Read the model definition and answer for the solid it produces. Units are mm, in the model's axes. Coordinates: 2 decimals unless noted, no trailing zeros. Write each loop counter-clockwise with the first axis right and the second up, starting at its lowest first coordinate (ties: lowest second). Pieces come first, ordered by that corner, then holes. Notation, with made-up numbers: M -38.75,27 L 19.25,27 A21 ccw 19.25,56 Z; hole C 61,25 d5. An arc over 180 degrees is marked long. Use a Markdown table: item, result. Add a question column.
from build123d import *

# Parameters (mm, degrees)
SKETCH1_R                  = 12.5
BOSS_EXTRUDE1_DEPTH        = 1.6002
F_10_CLEARANCE_HOLE1_D     = 4.9784
F_10_CLEARANCE_HOLE1_DEPTH = 172.97
F_10_CLEARANCE_HOLE1_TIP   = 1.495662253


with BuildPart() as part:
    # Sketch1 → Boss-Extrude1 (new body)
    with BuildSketch(Plane(origin=(0, 0, 0), x_dir=(1, 0, 0), z_dir=(0, 1, 0))):
        with BuildLine():
            ThreePointArc((-40, -34.7625), (-44.3084106, -32.029533038), (-43.672046889, -26.967265607))
            Line((-43.672046889, -26.967265607), (-12.722052212, 10.507111283))
            ThreePointArc((-12.722052212, 10.507111283), (0, 16.5), (12.722052212, 10.507111283))
            Line((12.722052212, 10.507111283), (43.672046889, -26.967265607))
            ThreePointArc((43.672046889, -26.967265607), (44.3084106, -32.029533038), (40, -34.7625))
            Line((40, -34.7625), (-40, -34.7625))
        make_face()
        with Locations(Location((0, 0, 0), (0, 0, 270))):  # turned: the seam where the file's is
            Circle(SKETCH1_R, mode=Mode.SUBTRACT)
    extrude(amount=BOSS_EXTRUDE1_DEPTH)

    # #10 Clearance Hole1
    with Locations(Plane(origin=(0, 1.6002, 0), x_dir=(1, 0, 0), z_dir=(0, 1, 0))):
        with Locations((40, -30), (-40, -30)):
            Hole(F_10_CLEARANCE_HOLE1_D / 2, depth=F_10_CLEARANCE_HOLE1_DEPTH)
            with Locations((0, 0, -(F_10_CLEARANCE_HOLE1_DEPTH + F_10_CLEARANCE_HOLE1_TIP / 2))):  # 118° drill point
                Cone(0, F_10_CLEARANCE_HOLE1_D / 2, F_10_CLEARANCE_HOLE1_TIP, mode=Mode.SUBTRACT)


solid = part.part
Item 1: Find section D-D on z = 0. Give the vertices of the cut face in (x, y).
Item 2: Each of these flat-tipped pins is pushed along its axis until it touches: pin 1 (15 mm diameter, centred on x = 0, z = 0, fed in from +Y); pin 2 (8 mm diameter, centred on x = 40, z = 30, fed in from -Y). Where does it stop, or does it pass through?
Item 3: Determine the mould class of faces 1 (the cylindrical face through (41.98, 0.79, 31.51)), 2 (the flat face through (1, 0, 20)), 3 (the flat face through (27.98, 0.79, 7.97)), 4 (the flat face through (1, 1, 34.762)) for opening direction Z: pulls with the +Z half, pulls with the -Z half, needs draft (parallel to the pull), parting line crosses it, or undercut.
Item 4: Find section C-C on z = 8.5. Give the vertices of the cut face in (x, y), then the cut area to 3 significant figures.
Item 5: Find section A-A on y = 0.3. Give the vertices of the cut face in (x, z) (1 decimal), then the cut area to 3 significant figures.
Item 6: Consider probe 1 along X at (y, z) = (1.1, 30); probe 2 along X at (y, z) = (0.7, 31); probe 3 along X at (y, z) = (1.4, 9.5). Determine where each line is inside the solid, lowest interval first.
Item 7: Find section B-B on z = 30. Give the vertices of the cut face in (x, y).
Geometry says:
| question | item | result |
|---|---|---|
| 1 | outline | M -21.4,0 L -12.5,0 L -12.5,1.6 L -21.4,1.6 Z; M 12.5,0 L 21.4,0 L 21.4,1.6 L 12.5,1.6 Z |
| 2 | pin 1 | passes through |
| 2 | pin 2 | stops at y = 0 |
| 3 | face 1 | undercut |
| 3 | face 2 | needs draft |
| 3 | face 3 | pulls with the -Z half |
| 3 | face 4 | pulls with the +Z half |
| 4 | outline | M -28.42,0 L -9.17,0 L -9.17,1.6 L -28.42,1.6 Z; M 9.17,0 L 28.42,0 L 28.42,1.6 L 9.17,1.6 Z |
| 4 | area | 61.6 mm2 |
| 5 | outline | M -43.7,27 L -12.7,-10.5 A16.5 ccw 12.7,-10.5 L 43.7,27 A4.8 ccw 40,34.8 L -40,34.8 A4.8 ccw Z; hole C -40,30 d5; hole C 0,0 d25; hole C 40,30 d5 |
| 5 | area | 2,380 mm2 |
| 6 | probe 1 | x = -44.76 to -42.49, -37.51 to 37.51, 42.49 to 44.76 |
| 6 | probe 2 | x = -44.66 to -42.28, -37.72 to 37.72, 42.28 to 44.66 |
| 6 | probe 3 | x = -29.25 to -8.12, 8.12 to 29.25 |
| 7 | outline | M -44.76,0 L -42.49,0 L -42.49,1.6 L -44.76,1.6 Z; M -37.51,0 L 37.51,0 L 37.51,1.6 L -37.51,1.6 Z; M 42.49,0 L 44.76,0 L 44.76,1.6 L 42.49,1.6 Z |
